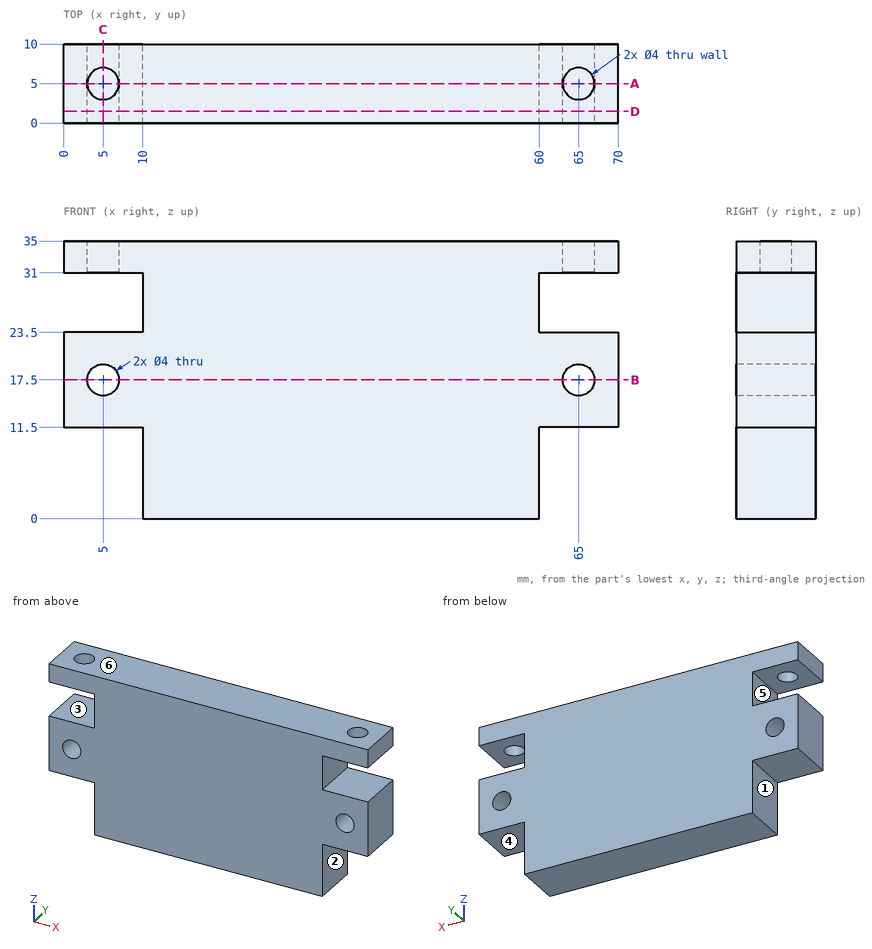
Input: dimensioned drawing with shaded views. Units: mm. Origin: part minimum x, y, z. A direction names the side the tool comes from. Give positions to 0.01 mm unless a question says otherwise; leave off trailing zeros. Write each loop counter-clockwise with the first axis right and the second up, starting at its lowest first coordinate (ties: lowest second). Pieces come first, ordered by that corner, then holes.
1. Reachability of the marked faces 1, 2 and 3 from +Z, -Z, +X, -X, +Y, -Y: full face, straight path, thin tool, end or side. Return the list, or none.
2. Line query: probe 1 along Y at (x, z) = (65, 33); probe 2 along Z at (x, y) = (65, 6.75); probe 3 along Z at (x, y) = (8, 2.25). Output: solid intervals per line, ascending.
3. Section query C-C, the plane x = 5. Return loops of the section in (y, z), then the cut area to 3 significant figures.
4. Draft query along Z for the marked faces 4, 5 and 6. Return one class per face: released by +Z, released by -Z, zero draft, split by the parting line, or undercut.
5. Section query B-B, the plane z = 17.5. Return loops of the section in (x, y), then the cut area to 3 significant figures.
6. Section query A-A, the plane y = 5. Return loops of the section in (x, z), then the cut area to 3 significant figures.
7. Pin query (flat end, axial travel): P1, Ø3, axis at y = 3, z = 4, coming from the +X side; P2, Ø3, axis at x = 66, y = 6, coming from the -Z side; P3, Ø3, axis at y = 4.5, z = 8, coming from the -X side. Return the tip coordinate at first contact, or that it passes through.
8. Section query D-D, the plane y = 1.5. Return loops of the section in (x, z).
Computed:
1. face 1: -Z, -X, +Y, -Y
1. face 2: -Z, +X, +Y, -Y
1. face 3: -X, +Y, -Y
2. probe 1: y = 0 to 3, 7 to 10
2. probe 2: z = 11.5 to 15.5, 19.5 to 23.5
2. probe 3: z = 11.5 to 23.5, 31 to 35
3. outline: (0, 11.5) - (10, 11.5) - (10, 15.5) - (0, 15.5) - close; (0, 19.5) - (10, 19.5) - (10, 23.5) - (0, 23.5) - close; (0, 31) - (3, 31) - (3, 35) - (0, 35) - close; (7, 31) - (10, 31) - (10, 35) - (7, 35) - close
3. area: 104 mm2
4. face 4: released by -Z
4. face 5: undercut
4. face 6: released by +Z
5. outline: (0, 0) - (3, 0) - (3, 10) - (0, 10) - close; (7, 0) - (63, 0) - (63, 10) - (7, 10) - close; (67, 0) - (70, 0) - (70, 10) - (67, 10) - close
5. area: 620 mm2
6. outline: (0, 11.5) - (10, 11.5) - (10, 0) - (60, 0) - (60, 11.5) - (70, 11.5) - (70, 23.5) - (60, 23.5) - (60, 31) - (63, 31) - (63, 35) - (7, 35) - (7, 31) - (10, 31) - (10, 23.5) - (0, 23.5) - close; (0, 31) - (3, 31) - (3, 35) - (0, 35) - close; (67, 31) - (70, 31) - (70, 35) - (67, 35) - close; hole circle Ø4 at (5, 17.5); hole circle Ø4 at (65, 17.5)
6. area: 2,010 mm2
7. P1: stops at x = 60
7. P2: stops at z = 11.5
7. P3: stops at x = 10
8. outline: (0, 11.5) - (10, 11.5) - (10, 0) - (60, 0) - (60, 11.5) - (70, 11.5) - (70, 23.5) - (60, 23.5) - (60, 31) - (70, 31) - (70, 35) - (0, 35) - (0, 31) - (10, 31) - (10, 23.5) - (0, 23.5) - close; hole circle Ø4 at (5, 17.5); hole circle Ø4 at (65, 17.5)
